```python
from build123d import *

# Parameters (mm, degrees)
BOX_W     = 30
BOX_H     = 8
BOX_DEPTH = 2
PAD_DEPTH = 20


with BuildPart() as cube:
    # Box → Box (new body)
    with BuildSketch(Plane(origin=(-15, -14, -1), x_dir=(1, 0, 0), z_dir=(0, 0, 1))):
        with Locations((15, 4)):
            Rectangle(BOX_W, BOX_H)
    extrude(amount=BOX_DEPTH)


with BuildPart() as cut:
    # Sketch001 → Pad (new body)
    with BuildSketch(Plane.XZ):
        with BuildLine():
            ThreePointArc((4.254276, 1.593075), (0.107321, 4.541501), (-4.174276, 1.792251))
            ThreePointArc((-4.903411, 1.857822), (-4.556737, 1.626068), (-4.174276, 1.792251))
            ThreePointArc((-4.903411, 1.857822), (-13.456487, -0.068818), (-4.848247, -1.731724))
            ThreePointArc((-4.141644, -1.811432), (-4.474352, -1.589018), (-4.848247, -1.731724))
            ThreePointArc((-4.141644, -1.811432), (-0.029723, -4.520356), (4.117465, -1.865739))
            ThreePointArc((4.873323, -1.837964), (4.486531, -1.610669), (4.117465, -1.865739))
            ThreePointArc((4.873323, -1.837964), (13.505182, 0.115954), (4.784336, 1.623809))
            ThreePointArc((4.254276, 1.593075), (4.524261, 1.522978), (4.784336, 1.623809))
        make_face()
        with BuildLine():
            ThreePointArc((3.875197, 1.610758), (-0.003981, 4.196626), (-3.878246, 1.603403))
            ThreePointArc((-5.168346, 1.619355), (-4.527466, 1.274089), (-3.878246, 1.603403))
            ThreePointArc((-5.168346, 1.619355), (-13.118412, 0.002733), (-5.170487, -1.624384))
            ThreePointArc((-3.861033, -1.649724), (-4.508513, -1.262573), (-5.170487, -1.624384))
            ThreePointArc((-3.861033, -1.649724), (-0.044432, -4.198474), (3.825254, -1.731068))
            ThreePointArc((5.156586, -1.685491), (4.476572, -1.289173), (3.825254, -1.731068))
            ThreePointArc((5.156586, -1.685491), (13.185859, 0.025154), (5.136633, 1.639308))
            ThreePointArc((3.875197, 1.610758), (4.5143, 1.254541), (5.136633, 1.639308))
        make_face(mode=Mode.SUBTRACT)
    extrude(amount=PAD_DEPTH)

    # Cut: cut Cube
    add(cube.part, mode=Mode.SUBTRACT)


solid = cut.part
```
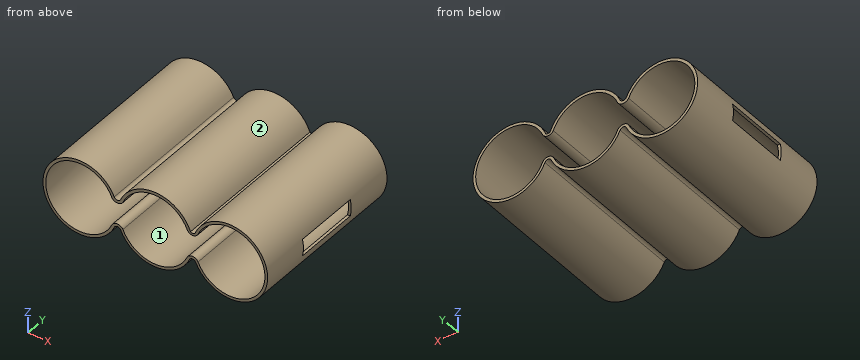
Check sheet for the modelled part. Datum: model origin and axes. Units: mm. Face numbers are marked on the shaded views. A direction names the side the tool comes from. Round coordinates to 2 decimals unless told otherwise and drop trailing zeros. Order: outer loops, then holes, each group sorted by start corner. A loop starts at its lowest first (then second) coordinate and runs counter-clockwise, first axis right, second up. Notation, with made-up numbers: M -32,87 L 11,87 A25 ccw 11,111 Z; hole C 74,-20.5 d7. An arc over 180 degrees is marked long. Answer in a Markdown table with one row per item.
(1) Gauge pin test, flat end, axial feed: pin 1 (3 mm diameter, centred on x = -7.5, y = -9, fed in from +Z). Record the tip position at first contact, or that the pin passes through.
Findings:
| item | result |
|---|---|
| pin 1 | stops at z = 4.48 |
(2) Section check C-C on z = -3.5. Record the boundary of the cut face in (x, y).
Findings:
| item | result |
|---|---|
| outline | M -11.77,-20 L -11.19,-20 L -11.19,0 L -11.77,0 Z; M -6.77,-20 L -6.18,-20 L -6.18,0 L -6.77,0 Z; M -2.86,-20 L -2.32,-20 L -2.32,0 L -2.86,0 Z; M 2.32,-20 L 2.86,-20 L 2.86,0 L 2.32,0 Z; M 6.15,-20 L 6.69,-20 L 6.69,0 L 6.15,0 Z; M 11.3,-20 L 11.84,-20 L 11.84,0 L 11.3,0 Z |
(3) Set-up check for the marked faces 1 and 2: record each of +Z, -Z, +X, -X, +Y, -Y from which the full face is reachable in a straight line by a thin tool's end or side.
Findings:
| item | result |
|---|---|
| face 1 | +Y, -Y |
| face 2 | +Z, +Y, -Y |
(4) Material ranges on line 1 along X through (y, z) = (-14.5, 1); line 2 along X through (y, z) = (-10.5, 2.25); line 3 along X through (y, z) = (-17.25, 3.75), recorded low to high. Write a range as from..to.
Findings:
| item | result |
|---|---|
| line 1 | x = -13.34..-13, 13.06..13.39 |
| line 2 | x = -12.85..-12.45, -5.5..-5.11, -3.95..-3.54, 3.54..3.95, 5.08..5.46, 12.53..12.91 |
| line 3 | x = -11.43..-10.73, -7.22..-6.53, -2.56..-1.88, 1.88..2.56, 6.48..7.12, 10.87..11.5 |
(5) Section check B-B on x = 6. Record the boundary of the cut face in (y, z).
Findings:
| item | result |
|---|---|
| outline | M -20,-3.38 L 0,-3.38 L 0,-2.93 L -20,-2.93 Z; M -20,2.93 L 0,2.93 L 0,3.38 L -20,3.38 Z |
(6) Section check D-D on y = -11. Record the boundary of the cut face in (x, z).
Findings:
| item | result |
|---|---|
| outline | M -13.34,-1 A4.48 ccw -4.85,-1.73 A0.44 cw -4.14,-1.81 A4.52 ccw 4.12,-1.87 A0.42 cw 4.87,-1.84 A4.51 ccw 13.39,-1 L 13.06,-1 A4.19 cw 5.16,-1.69 A0.74 ccw 3.83,-1.73 A4.2 cw -3.86,-1.65 A0.76 ccw -5.17,-1.62 A4.14 cw -13,-1 Z; M -13.34,1 L -13,1 A4.14 cw -5.17,1.62 A0.79 ccw -3.88,1.6 A4.2 cw 3.88,1.61 A0.72 ccw 5.14,1.64 A4.19 cw 13.06,1 L 13.39,1 A4.51 ccw 4.78,1.62 A0.45 cw 4.25,1.59 A4.54 ccw -4.17,1.79 A0.44 cw -4.9,1.86 A4.48 ccw Z |
(7) Section check A-A on z = 0. Record the boundary of the cut face in (x, y).
Findings:
| item | result |
|---|---|
| outline | M -13.46,-20 L -13.12,-20 L -13.12,-14 L -13.46,-14 Z; M -13.46,-6 L -13.12,-6 L -13.12,0 L -13.46,0 Z; M 13.19,-20 L 13.51,-20 L 13.51,-14 L 13.19,-14 Z; M 13.19,-6 L 13.51,-6 L 13.51,0 L 13.19,0 Z |
